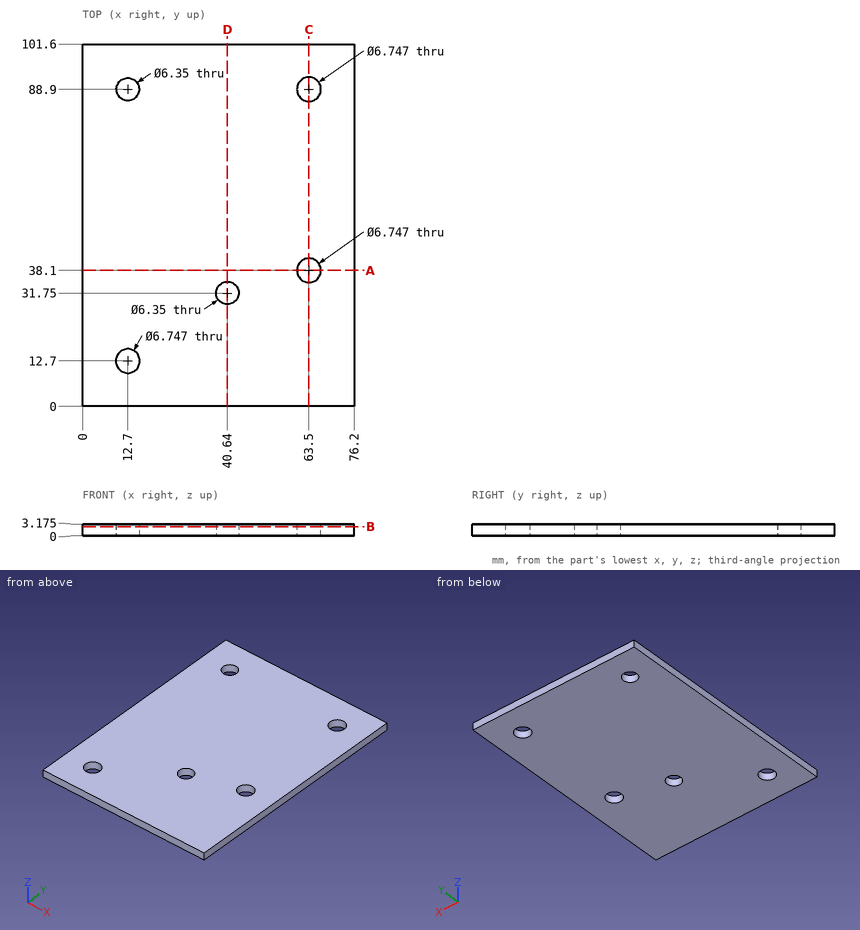
Verification items for this drawing (mm, ordinates from the low corner). Round coordinates to 2 decimals unless told otherwise and drop trailing zeros. Loops run counter-clockwise (first coordinate to the right, second up) from the corner with the lowest first, then second, coordinate; pieces in that order, holes last. Notation, with made-up numbers: (18, 80.5) - (43, 80.5) arc R28 cw to (43, 109.5) - close; hole circle Ø5 at (64.5, 39.5). An arc over 180 degrees is marked (long way). Answer as CSV lines item,"result". Start each with the question number.
Item 1: Scan lines: line 1 (Y direction, x = 63.5, z = 0.7); line 2 (X direction, y = 31.75, z = 1.8) (3 decimals); line 3 (X direction, y = 11.5, z = 0.45). Record each from-to range of solid material in increasing order. Write a range as [from, to].
Item 2: Section check A-A (y = 38.1). Record the boundary of the cut face in (x, z) (1 decimal).
Item 3: Section check C-C (x = 63.5). Record the boundary of the cut face in (y, z) (1 decimal).
Item 4: Section check B-B (z = 2.5). Count the separate pieces of the cut face and the enclosed holes in it, and give its area (3 significant figures).
Item 5: Section check D-D (x = 40.64). Record the boundary of the cut face in (y, z) (3 decimals).
Report:
1,line 1,"y = [0, 34.73], [41.47, 85.53], [92.27, 101.6]"
1,line 2,"x = [0, 37.465], [43.815, 76.2]"
1,line 3,"x = [0, 9.55], [15.85, 76.2]"
2,outline,"(0, 0) - (60.1, 0) - (60.1, 3.2) - (0, 3.2) - close; (66.9, 0) - (76.2, 0) - (76.2, 3.2) - (66.9, 3.2) - close"
3,outline,"(0, 0) - (34.7, 0) - (34.7, 3.2) - (0, 3.2) - close; (41.5, 0) - (85.5, 0) - (85.5, 3.2) - (41.5, 3.2) - close; (92.3, 0) - (101.6, 0) - (101.6, 3.2) - (92.3, 3.2) - close"
4,separate pieces,"1"
4,enclosed holes,"5"
4,area,"7,570 mm2"
5,outline,"(0, 0) - (28.575, 0) - (28.575, 3.175) - (0, 3.175) - close; (34.925, 0) - (101.6, 0) - (101.6, 3.175) - (34.925, 3.175) - close"
